```python
from build123d import *

# Parameters (mm, degrees)
SKETCH1_W           = 490
SKETCH1_H           = 210.49
BOSS_EXTRUDE1_DEPTH = 6
SKETCH2_W           = 6
SKETCH2_H           = 55.25
CUT_EXTRUDE1_DEPTH  = 534.331079256
SKETCH3_W           = 6
SKETCH3_H           = 91.92
CUT_EXTRUDE2_DEPTH  = 534.331079256
CUT_EXTRUDE3_DEPTH  = 534.331079256


with BuildPart() as part:
    # Sketch1 → Boss-Extrude1 (new body)
    with BuildSketch(Plane(origin=(0, 0, 0), x_dir=(1, 0, 0), z_dir=(0, 1, 0))):
        with Locations((245, 105.245)):
            Rectangle(SKETCH1_W, SKETCH1_H)
    extrude(amount=BOSS_EXTRUDE1_DEPTH)

    # Sketch2 → Cut-Extrude1 (cut, through all)
    with BuildSketch(Plane(origin=(0, 6, 0), x_dir=(1, 0, 0), z_dir=(0, 1, 0))):
        Polygon((411.666666663, 6), (411.666666663, 0), (490, 0), (490, 49.25), (484, 49.25), (484, 6), align=None)
        Polygon((0, 49.25), (0, 0), (78.33333333, 0), (78.33333333, 6), (6, 6), (6, 49.25), align=None)
        with Locations((487, 182.865)):
            Rectangle(SKETCH2_W, SKETCH2_H)
        with Locations((3, 182.865)):
            Rectangle(SKETCH2_W, SKETCH2_H)
    extrude(amount=-CUT_EXTRUDE1_DEPTH, mode=Mode.SUBTRACT)

    # Sketch3 → Cut-Extrude2 (cut, through all)
    with BuildSketch(Plane(origin=(0, 6, 0), x_dir=(1, 0, 0), z_dir=(0, 1, 0))):
        with Locations((245, 95.96)):
            Rectangle(SKETCH3_W, SKETCH3_H)
    extrude(amount=-CUT_EXTRUDE2_DEPTH, mode=Mode.SUBTRACT)

    # Sketch4 → Cut-Extrude3 (cut, through all)
    with BuildSketch(Plane(origin=(0, 6, 0), x_dir=(1, 0, 0), z_dir=(0, 1, 0))):
        with BuildLine():
            Line((119, 210.49), (119, 201.74))
            ThreePointArc((119, 201.74), (125.25, 195.49), (131.5, 201.74))
            Line((131.5, 201.74), (131.5, 210.49))
            Line((131.5, 210.49), (119, 210.49))
        make_face()
    extrude(amount=-CUT_EXTRUDE3_DEPTH, mode=Mode.SUBTRACT)


solid = part.part
```
Check sheet for the modelled part. Datum: model origin and axes. Units: mm. Round coordinates to 2 decimals unless told otherwise and drop trailing zeros. Loops run counter-clockwise (first coordinate to the right, second up) from the corner with the lowest first, then second, coordinate; pieces in that order, holes last. Notation, with made-up numbers: M 40.25,12 L 94.25,12 A15 ccw 94.25,19 Z; hole C 87.25,31 d4. An arc over 180 degrees is marked long. Answer as a JSON object with one key per item and string values.
1. Section check C-C (x = 455.5). Record the boundary of the cut face in (y, z).
Reply:
{"outline": "M 0,-210.49 L 6,-210.49 L 6,-6 L 0,-6 Z"}
2. Section check A-A (y = 2.1). Record the boundary of the cut face in (x, z), plus the area to 3 significant figures.
Reply:
{"outline": "M 0,-155.24 L 6,-155.24 L 6,-210.49 L 119,-210.49 L 119,-201.74 A6.25 cw 131.5,-201.74 L 131.5,-210.49 L 484,-210.49 L 484,-155.24 L 490,-155.24 L 490,-49.25 L 484,-49.25 L 484,-6 L 411.67,-6 L 411.67,0 L 78.33,0 L 78.33,-6 L 6,-6 L 6,-49.25 L 0,-49.25 Z; hole M 242,-141.92 L 248,-141.92 L 248,-50 L 242,-50 Z", "area": "100,000 mm²"}
3. Section check B-B (x = 125.25). Record the boundary of the cut face in (y, z).
Reply:
{"outline": "M 0,-195.49 L 6,-195.49 L 6,0 L 0,0 Z"}
4. Gauge pin test, flat ends, axial feed: P1, Ø4, axis at x = 411.5, z = -137.5, coming from the -Y side; P2, Ø1.8, axis at y = 1.5, z = -171, coming from the -X side; P3, Ø1.8, axis at x = 487, y = 3, coming from the +Z side; P4, Ø1.8, axis at y = 3, z = -2, coming from the -X side. Record the tip position at first contact, or that the pin passes through.
Reply:
{"P1": "stops at y = 0", "P2": "stops at x = 6", "P3": "stops at z = -49.25", "P4": "stops at x = 78.33"}
5. Scan lines: line 1 (X direction, y = 1, z = -136.5); line 2 (Z direction, x = 420, y = 2.35); line 3 (X direction, y = 3.65, z = -27.5). Record each from-to range of solid material in increasing order.
Reply:
{"line 1": "x = 0 to 242, 248 to 490", "line 2": "z = -210.49 to -6", "line 3": "x = 6 to 484"}
